Check sheet for the modelled part. Datum: model origin and axes. Units: mm. A direction names the side the tool comes from. Give positions to 0.01 mm unless a question says otherwise; leave off trailing zeros. Order: outer loops, then holes, each group sorted by start corner. A loop starts at its lowest first (then second) coordinate and runs counter-clockwise, first axis right, second up.
Item 1: Access from +Z, -Z, +X, -X, +Y, -Y to the whole of each face (thin tool, end or side, straight path). Record for faces 4 (the flat face through (9, -1.5, 19)), 5 (the flat face through (12, -19, 1)), 6 (the flat face through (12, 19, 1)), 7 (the cylindrical face through (12, 29, -29)).
Item 2: Sectioned sample at C-C on x = 12. Record the boundary of the cut face in (y, z).
Item 3: Release check for a two-part mould opening along Z. For faces 1 (the cylindrical face through (11.83, 0.53, -12.49)), 2 (the flat face through (12, 10, 25)), 3 (the flat face through (9, 1.5, 19)) record: released by +Z, released by -Z, zero draft, split by the parting line, or undercut.
Item 4: Gauge pin test, flat ends, axial feed: P1, Ø10, axis at x = 16, z = 16.5, coming from the -Y side; P2, Ø6.5, axis at x = 13.5, z = 20, coming from the +Y side; P3, Ø5, axis at x = 12, y = -27, coming from the +Z side. Record the tip position at first contact, or that the pin passes through.
Item 5: Material ranges on line 1 along Y through (x, z) = (12, -28); line 2 along Y through (x, z) = (14.75, 0); line 3 along Z through (x, y) = (12, 6), recorded low to high.
Item 6: Sectioned sample at A-A on z = 0. Record the boundary of the cut face in (x, y).
Item 7: Sectioned sample at B-B on y = -27. Record the boundary of the cut face in (x, z).
Item 8: Sectioned sample at D-D on x = 4.75. Record the boundary of the cut face in (y, z), and give its area (3 significant figures).
from build123d import *

# Parameters (mm, degrees)
BOSS_EXTRUDE1_DEPTH = 24
SKETCH2_R           = 2
CUT_EXTRUDE1_DEPTH  = 20
SKETCH3_R           = 2
CUT_EXTRUDE2_DEPTH  = 20.5


with BuildPart() as part:
    # Sketch1 → Boss-Extrude1 (new body)
    with BuildSketch(Plane(origin=(0, 0, 0), x_dir=(0, 0, -1), z_dir=(1, 0, 0))):
        with BuildLine():
            Line((23, 35), (23, 19))
            Line((23, 19), (-25, 19))
            Line((-25, 19), (-25, 1.5))
            Line((-25, 1.5), (-12.409673646, 1.5))
            ThreePointArc((-12.409673646, 1.5), (12.5, 0), (-12.409673646, -1.5))
            Line((-12.409673646, -1.5), (-25, -1.5))
            Line((-25, -1.5), (-25, -19))
            Line((-25, -19), (23, -19))
            Line((23, -19), (23, -35))
            Line((23, -35), (35, -35))
            Line((35, -35), (35, 35))
            Line((35, 35), (23, 35))
        make_face()
    extrude(amount=BOSS_EXTRUDE1_DEPTH)

    # Sketch2 → Cut-Extrude1 (cut)
    with BuildSketch(Plane.XY.offset(-23)):
        with Locations((12, -27)):
            Circle(SKETCH2_R)
    cut_extrude1 = extrude(amount=-CUT_EXTRUDE1_DEPTH, mode=Mode.SUBTRACT)

    # Sketch3 → Cut-Extrude2 (cut)
    with BuildSketch(Plane.XZ.offset(19)):
        with Locations(Location((12, 18.704836823, 0), (0, 0, 270))):
            Circle(SKETCH3_R)
    cut_extrude2 = extrude(amount=-CUT_EXTRUDE2_DEPTH, mode=Mode.SUBTRACT)

    # Mirror1: Cut-Extrude1, Cut-Extrude2 across plane
    add(cut_extrude1.mirror(Plane.ZX), mode=Mode.SUBTRACT)
    add(cut_extrude2.mirror(Plane.ZX), mode=Mode.SUBTRACT)


solid = part.part
Report:
1. face 4: +Z, +X, -X
1. face 5: +Z, +X, -X, -Y
1. face 6: +Z, +X, -X, +Y
1. face 7: +Z, -Z
2. outline: (-35, -35) - (-29, -35) - (-29, -23) - (-35, -23) - close; (-25, -35) - (25, -35) - (25, -23) - (19, -23) - (19, 16.7) - (1.5, 16.7) - (1.5, 12.41) arc R12.5 cw (long way) to (-1.5, 12.41) - (-1.5, 16.7) - (-19, 16.7) - (-19, -23) - (-25, -23) - close; (-19, 20.7) - (-1.5, 20.7) - (-1.5, 25) - (-19, 25) - close; (1.5, 20.7) - (19, 20.7) - (19, 25) - (1.5, 25) - close; (29, -35) - (35, -35) - (35, -23) - (29, -23) - close
3. face 1: undercut
3. face 2: released by +Z
3. face 3: zero draft
4. P1: stops at y = -19
4. P2: stops at y = 19
4. P3: stops at z = -23
5. line 1: y = -35 to -29, -25 to 25, 29 to 35
5. line 2: y = -19 to -12.5, 12.5 to 19
5. line 3: z = -35 to -10.97, 10.97 to 16.7, 20.7 to 25
6. outline: (0, -19) - (24, -19) - (24, -12.5) - (0, -12.5) - close; (0, 12.5) - (24, 12.5) - (24, 19) - (0, 19) - close
7. outline: (0, -35) - (10, -35) - (10, -23) - (0, -23) - close; (14, -35) - (24, -35) - (24, -23) - (14, -23) - close
8. outline: (-35, -35) - (35, -35) - (35, -23) - (19, -23) - (19, 25) - (1.5, 25) - (1.5, 12.41) arc R12.5 cw (long way) to (-1.5, 12.41) - (-1.5, 25) - (-19, 25) - (-19, -23) - (-35, -23) - close
8. area: 2,140 mm2
